CAD build for the part. Positions are in the model's coordinates, mm. Face numbers are marked on the shaded views. Round coordinates to 2 decimals unless told otherwise and drop trailing zeros. Loops run counter-clockwise (first coordinate to the right, second up) from the corner with the lowest first, then second, coordinate; pieces in that order, holes last. Notation, with made-up numbers: M 54.25,-6.75 L 68.25,-6.75 A25 cw 68.25,31.25 Z; hole C -31.5,-40 d9. An arc over 180 degrees is marked long. Put each result on its own line as item: value. Start each with the question number.
from build123d import *

# Parameters (mm, degrees)
F1_DEPTH      = 15
F1_DEPTH_BACK = 15
F3_DEPTH      = 19.001
F3_DEPTH_BACK = 21.001


with BuildPart() as f1:
    # F0 (on Top) → F1 (new body, two sides)
    with BuildSketch(Plane.XY) as f1_sk:
        Polygon((21, -25), (0, 20), (-15, 20), (-19, -21.1077940659), align=None)
    extrude(amount=F1_DEPTH)
    extrude(f1_sk.sketch, amount=-F1_DEPTH_BACK)

    # F2 (on Right) → F3 (cut, two sides)
    with BuildSketch(Plane.YZ) as f3_sk:
        with BuildLine():
            add(Edge.make_bspline(
                [(20, 4), (20, 15), (-5, 15)],
                knots=[0, 0, 0, 1.5707963268, 1.5707963268, 1.5707963268], degree=2, weights=[1, 0.7071067812, 1]))
            Line((20, 4), (20, 15))
            Line((20, 15), (-5, 15))
        make_face()
        with BuildLine():
            add(Edge.make_bspline(
                [(-5, -15), (20, -15), (20, -4)],
                knots=[4.7123889804, 4.7123889804, 4.7123889804, 6.2831853072, 6.2831853072, 6.2831853072], degree=2, weights=[1, 0.7071067812, 1]))
            Line((-5, -15), (20, -15))
            Line((20, -15), (20, -4))
        make_face()
    extrude(amount=-F3_DEPTH, mode=Mode.SUBTRACT)
    extrude(f3_sk.sketch, amount=F3_DEPTH_BACK, mode=Mode.SUBTRACT)


solid = f1.part
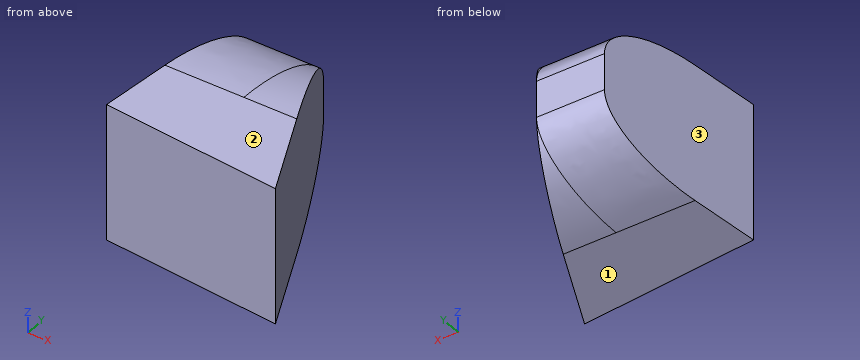
(1) Flat gauge pins, fed straight in: pin 1 Ø8 at (x, z) = (10.5, -6.5) entering from -Y; pin 2 Ø3 at (y, z) = (5, 4.5) entering from -X; pin 3 Ø2 at (y, z) = (-14, -11.5) entering from +X. Where does each tip first touch, or does it go through?
(2) Mould opens along Z. For the marked faces 1, 2 and 3 say: +Z half, -Z half, draft (parallel to the pull), parting line (faces both ways), or undercut.
(3) Drill centre lines: line 1 along X through (y, z) = (7, -13); line 2 along Y through (x, z) = (-12, 8); line 3 along Y through (x, z) = (-5, 8.5). Where is each one in solid material? Low to high.
(4) Cut at B-B on x = 13. List the corners of the cut face in (y, z), and give its area (3 significant figures).
(5) Cut at A-A on z = -1.5. List the corners of the cut face in (x, y), and give its area (3 significant figures).
Taken from the geometry:
1. pin 1: y = -24.37
1. pin 2: x = -16.61
1. pin 3: x = 16.33
2. face 1: -Z half
2. face 2: +Z half
2. face 3: draft
3. line 1: -16.26 to 6.07
3. line 2: -21.79 to 18.29
3. line 3: -22.47 to 17.81
4. outline: M -24.22,-15 L -7.86,-15 L -7.86,15 L -24.22,15 Z
4. area: 491 mm2
5. outline: M -19,-21.11 L 21,-25 L 0,20 L -15,20 Z
5. area: 1,170 mm2
